from build123d import *

# Parameters (mm, degrees)
F0_R     = 10
F0_R_2   = 6.35
F0_R_3   = 5.8166
F1_DEPTH = 5.08
F2_DEPTH = 23.368
F3_DEPTH = 42.418
F4_SIZE  = 1.27


with BuildPart() as f1:
    # F0 (on Top) → F1 (new body)
    with BuildSketch(Plane.XY):
        Circle(F0_R)
        Circle(F0_R_2, mode=Mode.SUBTRACT)
        Circle(F0_R_2)
        Circle(F0_R_3, mode=Mode.SUBTRACT)
        Circle(F0_R_3)
    extrude(amount=F1_DEPTH)

    # F0 (on Top) → F2 (join)
    with BuildSketch(Plane.XY):
        Circle(F0_R_2)
        Circle(F0_R_3, mode=Mode.SUBTRACT)
        Circle(F0_R_3)
    extrude(amount=F2_DEPTH)

    # F0 (on Top) → F3 (join)
    with BuildSketch(Plane.XY):
        Circle(F0_R_3)
    extrude(amount=F3_DEPTH)

    # F4
    f4_edges = [f1.edges().sort_by_distance(p)[0] for p in [
        (-5.8166, 0, 42.418),
    ]]
    chamfer(f4_edges, length=F4_SIZE)


solid = f1.part
Geometry check sheet. Reference: the model listing, model coordinates, mm. A direction names the side the tool comes from. Coordinates: 2 decimals unless noted, no trailing zeros. Order: outer loops, then holes, each group sorted by start corner. A loop starts at its lowest first (then second) coordinate and runs counter-clockwise, first axis right, second up. Notation, with made-up numbers: (84, 62.25) - (131, 62.25) arc R11 cw to (131, 78.25) - close; hole circle Ø8 at (4, 37). An arc over 180 degrees is marked (long way). One line per item, written item: value.
(1) Sectioned sample at D-D (z = 34). Enter the section's corners in (x, y).
Data:
outline: circle Ø11.63 at (0, 0)
(2) Sectioned sample at C-C (z = 15.5). Enter the section's corners in (x, y), and give its area (3 significant figures).
Data:
outline: circle Ø12.7 at (0, 0)
area: 127 mm^2
(3) Thickness scan on probe 1 along Z at (x, y) = (-6.5, -0.5); probe 2 along Z at (x, y) = (2.5, -5.75); probe 3 along Y at (x, z) = (4.25, 4.5). Record the ranges inside material, lowest first. Write a range as from..to.
Data:
probe 1: z = 0..5.08
probe 2: z = 0..23.37
probe 3: y = -9.05..9.05
(4) Access from +Z, -Z, +X, -X, +Y, -Y to the whole of each face (thin tool, end or side, straight path). Record for faces 1 (the face through (0, 0, 0)), 2 (the face through (-1.26, -5.68, 32.13)).
Data:
face 1: -Z, +X, -X, +Y, -Y
face 2: +Z
(5) Depth check by flat-ended pin: pin 1 Ø10 at (x, y) = (6.5, -3.5) entering from -Z; pin 2 Ø12 at (x, z) = (-3.5, 35) entering from +Y; pin 3 Ø8 at (y, z) = (-8, 26.5) entering from +X; pin 4 Ø2 at (y, z) = (4.5, 26.5) entering from +X. Enter the tip coordinate at first touch or a pass-through.
Data:
pin 1: stops at z = 0
pin 2: stops at y = 5.82
pin 3: stops at x = 4.22
pin 4: stops at x = 4.65
(6) Sectioned sample at A-A (x = 0). Enter the section's corners in (y, z).
Data:
outline: (-10, 0) - (10, 0) - (10, 5.08) - (6.35, 5.08) - (6.35, 23.37) - (5.82, 23.37) - (5.82, 41.15) - (4.55, 42.42) - (-4.55, 42.42) - (-5.82, 41.15) - (-5.82, 23.37) - (-6.35, 23.37) - (-6.35, 5.08) - (-10, 5.08) - close
